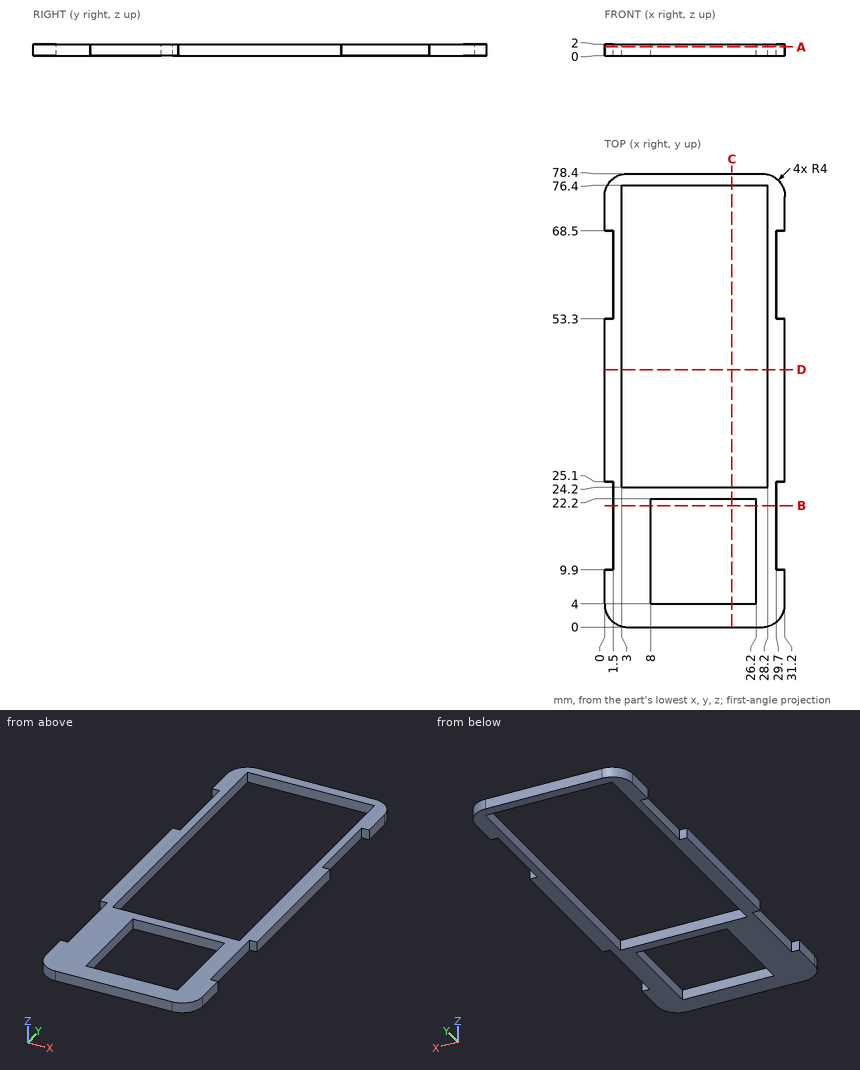
Study the drawing (mm; zero at the part's minimum x, y, z) and answer. Coordinates: 2 decimals unless noted, no trailing zeros. Order: outer loops, then holes, each group sorted by start corner. A loop starts at its lowest first (then second) coordinate and runs counter-clockwise, first axis right, second up. Notation, with made-up numbers: M -24.75,-20.5 L -5.75,-20.5 A27 cw -5.75,1.5 Z; hole C -34.75,-18.5 d10. An arc over 180 degrees is marked long. Answer as a JSON object with one key per item and string values. Group by question number.
1. Section A-A on z = 1.5 is taken. State how many separate pieces and enclosed holes the cut face has, then the cut area to 3 significant figures.
2. Section C-C on x = 22 is taken. Write down the section's boundary in (y, z).
3. Section D-D on y = 44.5 is taken. Write down the section's boundary in (x, z).
4. Section B-B on y = 21 is taken. Write down the section's boundary in (x, z).
5. Flat-ended cylindrical pins translate along their axes: P1, Ø0.8, axis at x = 1, z = 1, coming from the -Y side; P2, Ø1.2, axis at x = 0.5, z = 1, coming from the +Y side (3 decimals); P3, Ø1, axis at y = 17, z = 1.5, coming from the +X side. Find the tip coordinate at first contact, or state that the pin passes through.
6. Straight lines are drawn through the part: line 1 (Y direction, x = 25.5, z = 0.3); line 2 (X direction, y = 55.5, z = 1.65); line 3 (Y direction, x = 27, z = 0.35). For each, find the intervals that lie inside material, in ascending order.
Values follow:
{
 "1": {"separate pieces": "1", "enclosed holes": "2", "area": "694 mm2"},
 "2": {"outline": "M 0,0 L 4,0 L 4,2 L 0,2 Z; M 22.2,0 L 24.2,0 L 24.2,2 L 22.2,2 Z; M 76.4,0 L 78.4,0 L 78.4,2 L 76.4,2 Z"},
 "3": {"outline": "M 0,0 L 3,0 L 3,2 L 0,2 Z; M 28.2,0 L 31.2,0 L 31.2,2 L 28.2,2 Z"},
 "4": {"outline": "M 1.5,0 L 8,0 L 8,2 L 1.5,2 Z; M 26.2,0 L 29.7,0 L 29.7,2 L 26.2,2 Z"},
 "5": {"P1": "y = 0.96", "P2": "y = 77.155", "P3": "x = 29.7"},
 "6": {"line 1": "0 to 4, 22.2 to 24.2, 76.4 to 78.4", "line 2": "1.5 to 3, 28.2 to 29.7", "line 3": "0 to 24.2, 76.4 to 78.4"}
}
